Geometry: see drawing. Coordinates: mm, zero at the bounding-box minimum. A direction names the side the tool comes from. Coordinates: 2 decimals unless noted, no trailing zeros. Loops run counter-clockwise (first coordinate to the right, second up) from the corner with the lowest first, then second, coordinate; pieces in that order, holes last. Notation, with made-up numbers: M 22,30 L 41,30 A11 ccw 41,37 Z; hole C 51,47 d8. An arc over 180 degrees is marked long. One line per question, with ' | ' between items. Start each with the question number.
1. Ray query, probe 1 along Y at (x, z) = (118.03, 3); probe 2 along Y at (x, z) = (5, 7); probe 3 along X at (y, z) = (28, 5.75). Return the intervals inside material, ascending.
2. Pin query (flat end, axial travel): P1, Ø3, axis at x = 68.5, z = 6.5, coming from the -Y side. Return the tip coordinate at first contact, or that it passes through.
3. Access query for the marked faces 4, 5 and 6. Directions: +Z, -Z, +X, -X, +Y, -Y. A direction counts if a zero-diameter tool reaches every point of the face in a straight line with its end or side. Return the directions, or none.
4. Mould query, pull axis X, two halves, no side actions, for the marked faces 1, 2 and 3. Classes: pulls with the +X half, pulls with the -X half, needs draft (parallel to the pull), parting line crosses it, or undercut.
5. Section query C-C, the plane z = 3.5. Output: boundary loops of the cut face in (x, y).
6. Section query A-A, the plane x = 118.03. Output: boundary loops of the cut face in (y, z), and give its area (3 significant figures).
7. Section query B-B, the plane y = 55.8. Output: boundary loops of the cut face in (x, z), and give its area (3 significant figures).
8. Section query D-D, the plane y = 30.4. Output: boundary loops of the cut face in (x, z).
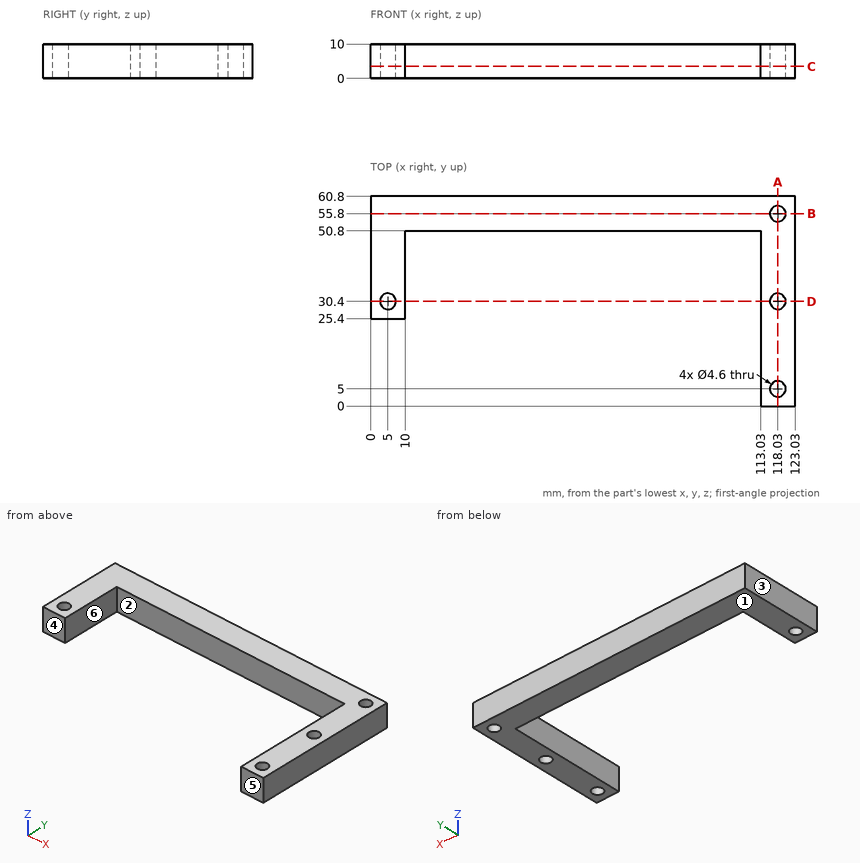
Taken from the geometry:
1) probe 1: 0 to 2.7, 7.3 to 28.1, 32.7 to 53.5, 58.1 to 60.8 | probe 2: 25.4 to 28.1, 32.7 to 60.8 | probe 3: 0 to 10, 113.03 to 123.03
2) P1: y = 50.8
3) face 4: +Z, -Z, -X, -Y | face 5: +Z, -Z, +X, -X, -Y | face 6: +Z, -Z, -Y
4) face 1: needs draft | face 2: undercut | face 3: pulls with the -X half
5) outline: M 0,25.4 L 10,25.4 L 10,50.8 L 113.03,50.8 L 113.03,0 L 123.03,0 L 123.03,60.8 L 0,60.8 Z; hole C 5,30.4 d4.6; hole C 118.03,5 d4.6; hole C 118.03,30.4 d4.6; hole C 118.03,55.8 d4.6
6) outline: M 0,0 L 2.7,0 L 2.7,10 L 0,10 Z; M 7.3,0 L 28.1,0 L 28.1,10 L 7.3,10 Z; M 32.7,0 L 53.5,0 L 53.5,10 L 32.7,10 Z; M 58.1,0 L 60.8,0 L 60.8,10 L 58.1,10 Z | area: 470 mm^2
7) outline: M 0,0 L 115.73,0 L 115.73,10 L 0,10 Z; M 120.33,0 L 123.03,0 L 123.03,10 L 120.33,10 Z | area: 1,180 mm^2
8) outline: M 0,0 L 2.7,0 L 2.7,10 L 0,10 Z; M 7.3,0 L 10,0 L 10,10 L 7.3,10 Z; M 113.03,0 L 115.73,0 L 115.73,10 L 113.03,10 Z; M 120.33,0 L 123.03,0 L 123.03,10 L 120.33,10 Z
